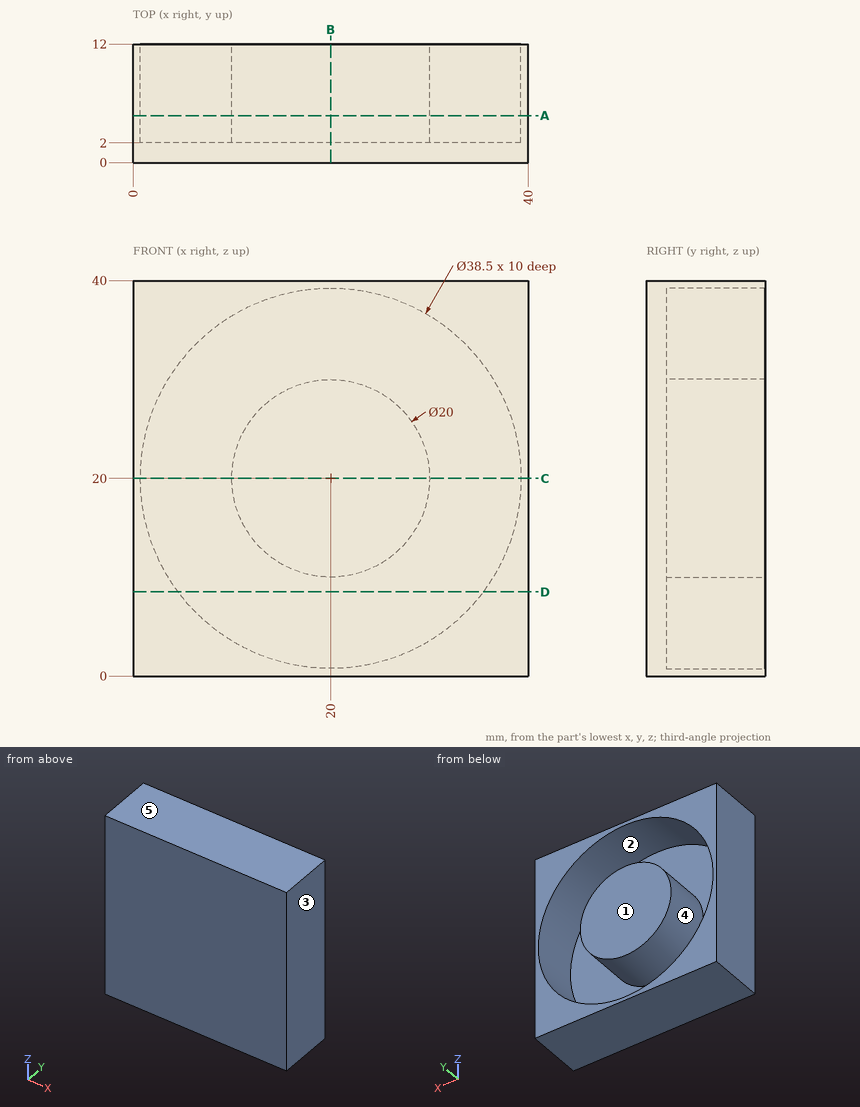
Drawing for the job (mm, zero at the part's lowest x, y, z). A direction names the side the tool comes from. Round coordinates to 2 decimals unless told otherwise and drop trailing zeros. Loops run counter-clockwise (first coordinate to the right, second up) from the corner with the lowest first, then second, coordinate; pieces in that order, holes last. Notation, with made-up numbers: (12, -5) -> (29, -5) arc R10 cw to (29, -1) -> close; hole circle Ø5 at (42.5, -22). An arc over 180 degrees is marked (long way). Answer as CSV lines item,"result". Start each with the question number.
1) Slice it at D-D (z = 8.5). List the corners of the cut face in (x, y).
2) Probe line 1 along X through (y, z) = (8.5, 20); line 2 along Z through (x, y) = (28, 5.5); line 3 along X through (y, z) = (3.5, 13.5). List the from-to ranges inside material, lowest first.
3) Slice it at B-B (x = 20). List the corners of the cut face in (y, z), plus the area to 3 significant figures.
4) Pin check, flat tip, straight feed: P1, Ø5, axis at x = 34, y = 5.5, coming from the -Z side. Stop position of the tip, or through.
5) Tool access for the marked faces 4 and 5: list every direction of +Z, -Z, +X, -X, +Y, -Y with a clear straight run to the whole face (end or side of a thin tool).
6) Slice it at A-A (y = 4.75). List the corners of the cut face in (x, z).
7) Slice it at C-C (z = 20). List the corners of the cut face in (x, y), plus the area to 3 significant figures.
8) Mould opens along X. For the marked faces 1, 2 and 3 say: +X half, -X half, draft (parallel to the pull), parting line (faces both ways), or undercut.
Filled in:
1,outline,"(0, 0) -> (40, 0) -> (40, 12) -> (35.44, 12) -> (35.44, 2) -> (4.56, 2) -> (4.56, 12) -> (0, 12) -> close"
2,line 1,"x = 0 to 0.75, 10 to 30, 39.25 to 40"
2,line 2,"z = 0 to 2.49, 14 to 26, 37.51 to 40"
2,line 3,"x = 0 to 1.88, 12.4 to 27.6, 38.12 to 40"
3,outline,"(0, 0) -> (12, 0) -> (12, 0.75) -> (2, 0.75) -> (2, 10) -> (12, 10) -> (12, 30) -> (2, 30) -> (2, 39.25) -> (12, 39.25) -> (12, 40) -> (0, 40) -> close"
3,area,"295 mm2"
4,P1,"stops at z = 0"
5,face 4,"+Y"
5,face 5,"+Z, +X, -X, +Y, -Y"
6,outline,"(0, 0) -> (40, 0) -> (40, 40) -> (0, 40) -> close; circle Ø20 at (20, 20); hole circle Ø38.5 at (20, 20)"
7,outline,"(0, 0) -> (40, 0) -> (40, 12) -> (39.25, 12) -> (39.25, 2) -> (30, 2) -> (30, 12) -> (10, 12) -> (10, 2) -> (0.75, 2) -> (0.75, 12) -> (0, 12) -> close"
7,area,"295 mm2"
8,face 1,"draft"
8,face 2,"undercut"
8,face 3,"+X half"
